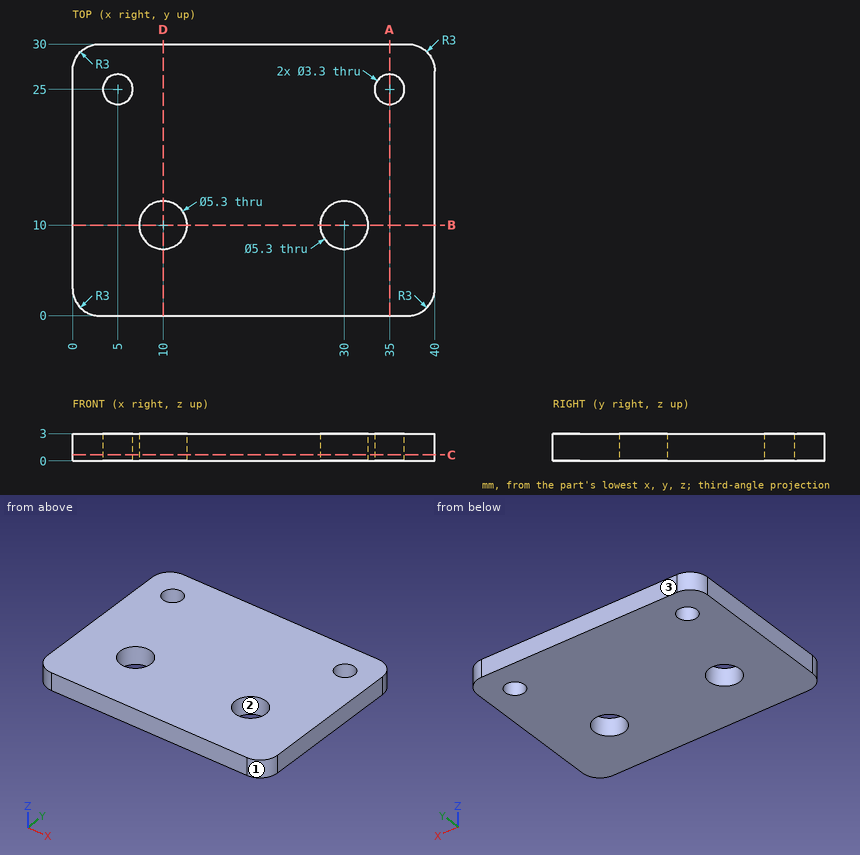
Input: dimensioned drawing with shaded views. Units: mm. Origin: part minimum x, y, z. Round coordinates to 2 decimals unless told otherwise and drop trailing zeros. Order: outer loops, then holes, each group sorted by start corner. A loop starts at its lowest first (then second) coordinate and runs counter-clockwise, first axis right, second up. Notation, with made-up numbers: (22.5, -14.75) - (36.5, -14.75) arc R10 cw to (36.5, 3.25) - close; hole circle Ø7 at (2, 43.25). An arc over 180 degrees is marked (long way). Write item = value, one per line. Start each with the question number.
Q1. Cut plane A-A on x = 35. Return the cut outline in (y, z).
Q2. Pull-direction query (X, two-part tool) for the marked faces 1, 2 and 3; classes: +X half, -X half, draft (parallel to the pull), parting line (faces both ways), or undercut.
Q3. Ray query, line 1 (Y direction, x = 30, z = 0.7); line 2 (X direction, y = 26, z = 0.3); line 3 (Y direction, x = 5, z = 1.3). Return the intervals inside material, ascending. Write a range as from..to.
Q4. Cut plane B-B on y = 10. Return the cut outline in (x, z).
Q5. Cut plane D-D on x = 10. Return the cut outline in (y, z).
Q6. Cut plane C-C on z = 0.65. Return the cut outline in (x, y).
Outcome:
q1.outline = (0, 0) - (23.35, 0) - (23.35, 3) - (0, 3) - close; (26.65, 0) - (30, 0) - (30, 3) - (26.65, 3) - close
q2.face_1 = +X half
q2.face_2 = undercut
q2.face_3 = draft
q3.line_1 = 0..7.35, 12.65..30
q3.line_2 = 0..3.69, 6.31..33.69, 36.31..40
q3.line_3 = 0..23.35, 26.65..30
q4.outline = (0, 0) - (7.35, 0) - (7.35, 3) - (0, 3) - close; (12.65, 0) - (27.35, 0) - (27.35, 3) - (12.65, 3) - close; (32.65, 0) - (40, 0) - (40, 3) - (32.65, 3) - close
q5.outline = (0, 0) - (7.35, 0) - (7.35, 3) - (0, 3) - close; (12.65, 0) - (30, 0) - (30, 3) - (12.65, 3) - close
q6.outline = (0, 3) arc R3 ccw to (3, 0) - (37, 0) arc R3 ccw to (40, 3) - (40, 27) arc R3 ccw to (37, 30) - (3, 30) arc R3 ccw to (0, 27) - close; hole circle Ø3.3 at (5, 25); hole circle Ø5.3 at (10, 10); hole circle Ø5.3 at (30, 10); hole circle Ø3.3 at (35, 25)
